Can you work these out from the model? Positions are in its coordinate system, mm. Face numbers are marked on the shaded views. Coordinates: 2 decimals unless noted, no trailing zeros. Write each loop counter-clockwise with the first axis right and the second up, starting at its lowest first coordinate (ties: lowest second). Pieces come first, ordered by that corner, then holes. Notation, with made-up numbers: (78.5, 1.25) - (102.5, 1.25) arc R19 ccw to (102.5, 25.25) - close; hole circle Ø1 at (9, 79). An arc over 180 degrees is marked (long way). Use one line per item in the form item = value. Start each with the question number.
(1) If we section it at A-A on y = -43.5: Give the number of separate pieces and of enclosed holes in the cut face, then the cut area to 3 significant figures.
(2) For pin 1 Ø1.5 at (x, z) = (0.5, 25.5) entering from -Y, with a flat end and sliding along its axis, tell me the tip position at first contact or that it passes through.
(3) If I drill on probe 1 along Y at (x, z) = (17.5, 26); probe 2 along Y at (x, z) = (12, -1.5); probe 3 along Z at (x, y) = (11.5, -3.5), over which ranges is the centre line in solid material (lowest first)? Write a range as from..to.
(4) If we section it at B-B on z = -45: Please give me the cut outline in (x, y).
(5) Thinking about a two-plate mould opening in X: for the marked faces 1, 2 and 3, which applies, pulls with the +X half, pulls with the -X half, needs draft (parallel to the pull), parting line crosses it, or undercut?
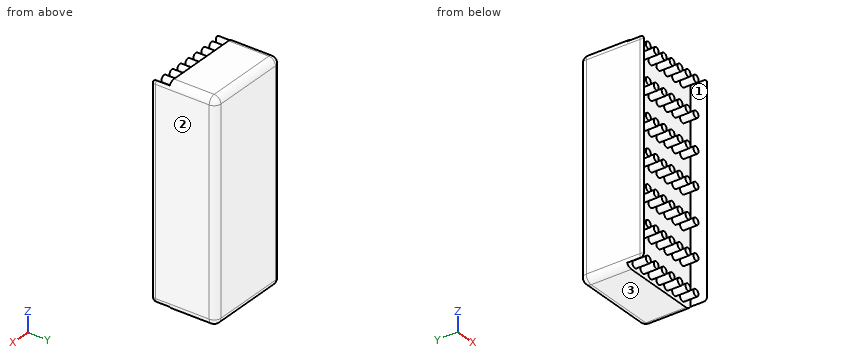
```python
from build123d import *

# Parameters (mm, degrees)
F0_W     = 65
F0_H     = 160
F1_DEPTH = 50
F2_R     = 5
F3_W     = 63.614636
F3_H     = 163.49268
F4_DEPTH = 15
F5_R     = 2.5
F6_DEPTH = 10


with BuildPart() as f1:
    # F0 (on Front) → F1 (new body)
    with BuildSketch(Plane.XZ):
        Rectangle(F0_W, F0_H)
    extrude(amount=F1_DEPTH)

    # F2
    f2_edges = [f1.edges().sort_by_distance(p)[0] for p in [
        (32.5, -25, 80),
        (-32.5, -25, 80),
        (0, 0, 80),
        (32.5, 0, 0),
        (32.5, -50, 0),
        (-32.5, -50, 0),
        (0, -50, -80),
        (32.5, -25, -80),
        (-32.5, -25, -80),
        (0, 0, -80),
        (-32.5, 0, 0),
        (0, -50, 80),
    ]]
    fillet(f2_edges, radius=F2_R)

    # F3 (on face) → F4 (cut)
    with BuildSketch(Plane.XZ.offset(50)):
        Rectangle(F3_W, F3_H)
    extrude(amount=-F4_DEPTH, mode=Mode.SUBTRACT)

    # F5 (on face) → F6 (join)
    with BuildSketch(Plane.XZ.offset(35)):
        Circle(F5_R)
        with Locations((0, 25)):
            Circle(F5_R)
        with Locations((0, 50)):
            Circle(F5_R)
        with Locations((0, 75)):
            Circle(F5_R)
        with Locations((8, 0)):
            Circle(F5_R)
        with Locations((8, 25)):
            Circle(F5_R)
        with Locations((8, 50)):
            Circle(F5_R)
        with Locations((8, 75)):
            Circle(F5_R)
        with Locations((16, 0)):
            Circle(F5_R)
        with Locations((16, 25)):
            Circle(F5_R)
        with Locations((16, 50)):
            Circle(F5_R)
        with Locations((16, 75)):
            Circle(F5_R)
        with Locations((24, 0)):
            Circle(F5_R)
        with Locations((24, 25)):
            Circle(F5_R)
        with Locations((24, 50)):
            Circle(F5_R)
        with Locations((24, 75)):
            Circle(F5_R)
        with Locations((-8, 0)):
            Circle(F5_R)
        with Locations((-24, 0)):
            Circle(F5_R)
        with Locations((-24, 25)):
            Circle(F5_R)
        with Locations((-16, 0)):
            Circle(F5_R)
        with Locations((-24, 50)):
            Circle(F5_R)
        with Locations((-16, 50)):
            Circle(F5_R)
        with Locations((-24, 75)):
            Circle(F5_R)
        with Locations((-8, 75)):
            Circle(F5_R)
        with Locations((-16, 25)):
            Circle(F5_R)
        with Locations((-8, 50)):
            Circle(F5_R)
        with Locations((-16, 75)):
            Circle(F5_R)
        with Locations((-8, 25)):
            Circle(F5_R)
        with Locations((0, -25)):
            Circle(F5_R)
        with Locations((0, -50)):
            Circle(F5_R)
        with Locations((0, -75)):
            Circle(F5_R)
        with Locations((16, -25)):
            Circle(F5_R)
        with Locations((16, -50)):
            Circle(F5_R)
        with Locations((-16, -25)):
            Circle(F5_R)
        with Locations((-8, -50)):
            Circle(F5_R)
        with Locations((24, -25)):
            Circle(F5_R)
        with Locations((-16, -75)):
            Circle(F5_R)
        with Locations((-24, -75)):
            Circle(F5_R)
        with Locations((8, -75)):
            Circle(F5_R)
        with Locations((24, -50)):
            Circle(F5_R)
        with Locations((-8, -25)):
            Circle(F5_R)
        with Locations((-24, -50)):
            Circle(F5_R)
        with Locations((8, -50)):
            Circle(F5_R)
        with Locations((24, -75)):
            Circle(F5_R)
        with Locations((-16, -50)):
            Circle(F5_R)
        with Locations((8, -25)):
            Circle(F5_R)
        with Locations((-24, -25)):
            Circle(F5_R)
        with Locations((-8, -75)):
            Circle(F5_R)
        with Locations((16, -75)):
            Circle(F5_R)
    extrude(amount=F6_DEPTH)


solid = f1.part
```
Reported:
q1.separate_pieces = 51
q1.enclosed_holes = 0
q1.area = 1,170 mm2
q2.pin_1 = -45
q3.probe_1 = -45..0
q3.probe_2 = -35..0
q3.probe_3 = -79.77..79.77
q4.outline = (-32.5, -45) arc R5 ccw to (-31.81, -47.54) - (-31.81, -35) - (31.81, -35) - (31.81, -47.54) arc R5 ccw to (32.5, -45) - (32.5, -5) arc R5 ccw to (27.5, 0) - (-27.5, 0) arc R5 ccw to (-32.5, -5) - close
q5.face_1 = undercut
q5.face_2 = pulls with the +X half
q5.face_3 = needs draft
